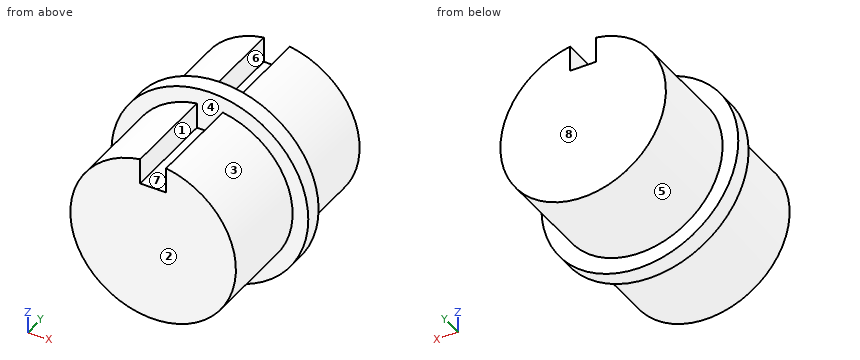
from build123d import *

# Parameters (mm, degrees)
F0_R     = 30.348394
F1_DEPTH = 38.1
F2_W     = 9.519064
F2_H     = 19.576774
F3_DEPTH = 101.6
F4_R     = 36.100393
F5_DEPTH = 3.175


with BuildPart() as f1:
    # F0 (on Front) → F1 (new body, symmetric)
    with BuildSketch(Plane.XZ):
        Circle(F0_R)
    extrude(amount=F1_DEPTH, both=True)

    # F2 (on face) → F3 (cut)
    with BuildSketch(Plane.XZ.offset(38.1)):
        with Locations((0, 30.348394)):
            Rectangle(F2_W, F2_H)
    extrude(amount=-F3_DEPTH, mode=Mode.SUBTRACT)

    # F4 (on Front) → F5 (join, symmetric)
    with BuildSketch(Plane.XZ):
        Circle(F4_R)
    extrude(amount=F5_DEPTH, both=True)


solid = f1.part
Model file for the job. Use its own axes, mm. Face numbers are marked on the shaded views. A direction names the side the tool comes from. Give positions to 0.01 mm unless a question says otherwise; leave off trailing zeros. Order: outer loops, then holes, each group sorted by start corner. A loop starts at its lowest first (then second) coordinate and runs counter-clockwise, first axis right, second up. Notation, with made-up numbers: M 2,-21 L 8,-21 A29 cw 8,3 Z; hole C 40.5,-11.75 d4. An arc over 180 degrees is marked long. Put each result on its own line as item: value. Start each with the question number.
(1) Drill centre lines: L1, parallel to Y at x = -7, z = -32 (3 decimals); L2, parallel to Z at x = 3, y = -18; L3, parallel to Z at x = -27.5, y = 27. Where is each one in solid material? Low to high. Write a range as [from, to].
(2) Band-saw the part on D-D on z = 24.5. Give the cut face in (x, y) (3 decimals).
(3) Band-saw the part on B-B on x = 0. Give the cut face in (y, z) (3 decimals).
(4) Band-saw the part on C-C on y = 17. Give the cut face in (x, z), then the cut area to 3 significant figures.
(5) Tool access for the marked faces 4, 5, 6, 7 and 8: list every direction of +Z, -Z, +X, -X, +Y, -Y with a clear straight run to the whole face (end or side of a thin tool).
(6) Pin check, flat tips, straight feed: pin 1 Ø1 at (x, y) = (0, 0.5) entering from -Z; pin 2 Ø2 at (x, y) = (20.5, -17.5) entering from +Z; pin 3 Ø3 at (y, z) = (13, 25.5) entering from -X. Stop position of each tip, or through.
(7) Band-saw the part on A-A on z = 0. Give the cut face in (x, y) (3 decimals), then the cut area to 3 significant figures.
(8) Pull direction X, two halves, no side cores. Call the marked faces 1, 2 and 3: released by +X, released by -X, zero draft, split by the parting line, or undercut.
Results below:
1. L1: y = [-3.175, 3.175]
1. L2: z = [-30.2, 20.56]
1. L3: z = [-12.84, 12.84]
2. outline: M -26.514,-3.175 L -17.91,-3.175 L -17.91,-38.1 L -4.76,-38.1 L -4.76,-3.175 L 4.76,-3.175 L 4.76,-38.1 L 17.91,-38.1 L 17.91,-3.175 L 26.514,-3.175 L 26.514,3.175 L 17.91,3.175 L 17.91,38.1 L 4.76,38.1 L 4.76,3.175 L -4.76,3.175 L -4.76,38.1 L -17.91,38.1 L -17.91,3.175 L -26.514,3.175 Z
3. outline: M -38.1,-30.348 L -3.175,-30.348 L -3.175,-36.1 L 3.175,-36.1 L 3.175,-30.348 L 38.1,-30.348 L 38.1,20.56 L 3.175,20.56 L 3.175,36.1 L -3.175,36.1 L -3.175,20.56 L -38.1,20.56 Z
4. outline: M -4.76,20.56 L -4.76,29.97 A30.35 ccw long 4.76,29.97 L 4.76,20.56 Z
4. area: 2,800 mm2
5. face 4: -Y
5. face 5: +Y
5. face 6: +Z, +Y
5. face 7: +Z, -Y
5. face 8: +Z, -Z, +X, -X, +Y
6. pin 1: stops at z = -36.1
6. pin 2: stops at z = 23.25
6. pin 3: stops at x = -18.57
7. outline: M -36.1,-3.175 L -30.348,-3.175 L -30.348,-38.1 L 30.348,-38.1 L 30.348,-3.175 L 36.1,-3.175 L 36.1,3.175 L 30.348,3.175 L 30.348,38.1 L -30.348,38.1 L -30.348,3.175 L -36.1,3.175 Z
7. area: 4,700 mm2
8. face 1: undercut
8. face 2: zero draft
8. face 3: split by the parting line
